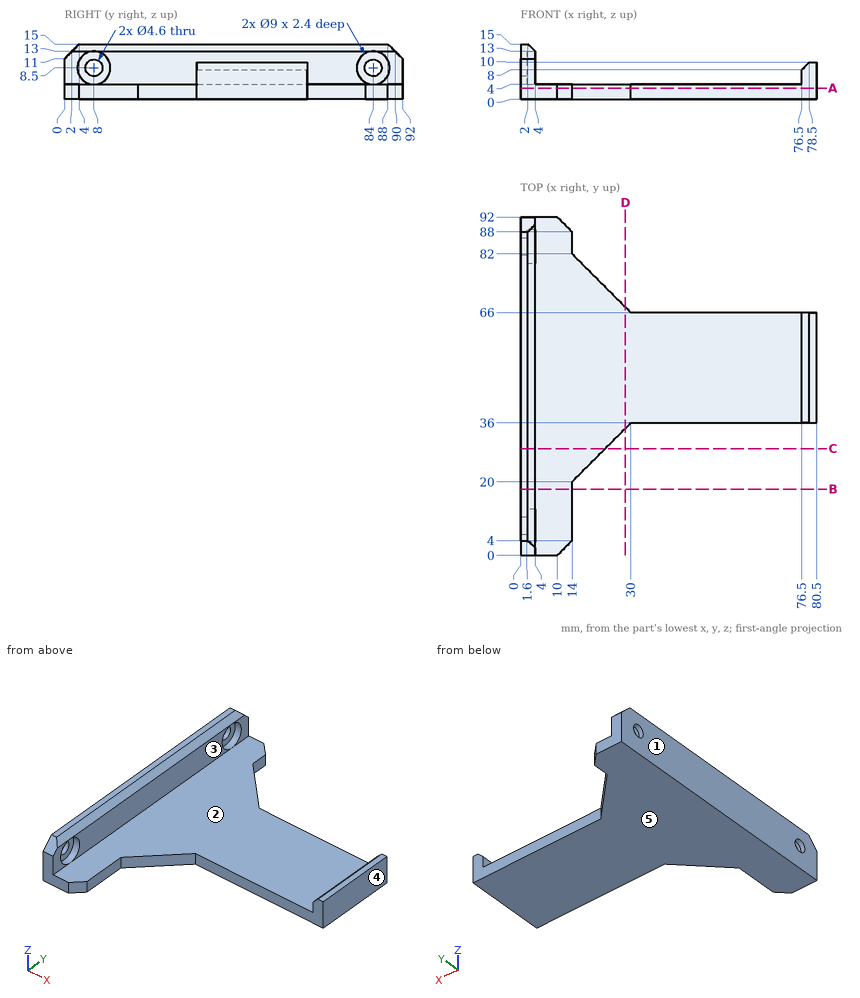
Geometry: see drawing. Coordinates: mm, zero at the bounding-box minimum. A direction names the side the tool comes from. Coordinates: 2 decimals unless noted, no trailing zeros. Write each loop counter-clockwise with the first axis right and the second up, starting at its lowest first coordinate (ties: lowest second). Pieces come first, ordered by that corner, then holes.
1) Section B-B on y = 18. Output: boundary loops of the cut face in (x, z), and give its area (3 significant figures).
2) Material intervals for line 1 along Z through (x, y) = (1, 84); line 2 along X through (y, z) = (81, 2); line 3 along X through (y, z) = (52, 10.25), sorted ascending.
3) Pin query (flat end, axial travel): pin 1 Ø0.6 at (x, y) = (79.5, 56.5) entering from +Z; pin 2 Ø8 at (x, z) = (44.5, 7.5) entering from -Y; pin 3 Ø1.5 at (y, z) = (12, 4.5) entering from +X. Return the tip coordinate at first contact, or that it passes through.
4) Section C-C on y = 29. Output: boundary loops of the cut face in (x, z), and give its area (3 significant figures).
5) Set-up query: the marked faces 1 and 2. Return all of +Z, -Z, +X, -X, +Y, -Y with unobstructed straight access to the full face (end or side cutting, diameter ignored); none if empty.
6) Section D-D on x = 28.5. Output: boundary loops of the cut face in (y, z).
7) Section A-A on z = 3. Output: boundary loops of the cut face in (x, y), and give its area (3 significant figures).
8) Mould query, pull axis X, two halves, no side actions, for the marked faces 3, 4 and 5. Classes: pulls with the +X half, pulls with the -X half, needs draft (parallel to the pull), parting line crosses it, or undercut.
Check result:
1. outline: (0, 0) - (14, 0) - (14, 4) - (4, 4) - (4, 13) - (2, 15) - (0, 15) - close
1. area: 98.0 mm2
2. line 1: z = 0 to 6.2, 10.8 to 15
2. line 2: x = 0 to 15
2. line 3: x = 0 to 4
3. pin 1: stops at z = 10
3. pin 2: stops at y = 36
3. pin 3: stops at x = 14
4. outline: (0, 0) - (23, 0) - (23, 4) - (4, 4) - (4, 13) - (2, 15) - (0, 15) - close
4. area: 134 mm2
5. face 1: +Z, -Z, -X, +Y, -Y
5. face 2: +Z, +Y, -Y
6. outline: (34.5, 0) - (67.5, 0) - (67.5, 4) - (34.5, 4) - close
7. outline: (0, 0) - (10, 0) - (14, 4) - (14, 20) - (30, 36) - (80.5, 36) - (80.5, 66) - (30, 66) - (14, 82) - (14, 88) - (10, 92) - (0, 92) - close
7. area: 3,520 mm2
8. face 3: undercut
8. face 4: pulls with the +X half
8. face 5: needs draft
